Autodesk Inventor part; units mm, degrees
ref_plane "YZ Plane" through (0, 0, 0) normal (1, 0, 0) x (0, 1, 0)
ref_plane "XZ Plane" through (0, 0, 0) normal (0, 1, 0) x (-1, 0, 0)
ref_plane "XY Plane" through (0, 0, 0) normal (0, 0, 1) x (1, 0, 0)
sketch "Sketch1" plane through (0, 0, 0) normal (0, 1, 0) x (-1, 0, 0)
  line L0 (5.5, 6.5) -> (-5.5, 6.5)
  line L1 (-5.5, 6.5) -> (-5.5, -6.5)
  line L2 (-5.5, -6.5) -> (5.5, -6.5)
  line L3 (5.5, -6.5) -> (5.5, 6.5)
  line L4 (0, -9.1) -> (0, 9.1)
  line L5 (-7.7, 0) -> (7.7, 0)
  point P0 (0, 0)
  dimension "d0" = 11
  dimension "d1" = 5.5
  dimension "d2" = 13
  dimension "d3" = 6.5
extrude "Extrusion1" add sketch "Sketch1" along normal blind 5
sketch "Sketch2" plane through (0, 5, 0) normal (0, 1, 0) x (1, 0, 0)
  line L0 (-5.5, -6.5) -> (5.5, -6.5)
  line L1 (-5.24, -6.5) -> (-4.24, -6.5)
  line L2 (-4.24, -6.5) -> (-4.24, 1)
  line L3 (-4.24, 1) -> (-5.24, 1)
  line L4 (-5.24, 1) -> (-5.24, -6.5)
  line L5 (5.24, -6.5) -> (4.24, -6.5)
  line L6 (4.24, -6.5) -> (4.24, 1)
  line L7 (4.24, 1) -> (5.24, 1)
  line L8 (5.24, 1) -> (5.24, -6.5)
  line L9 (5.5, -6.5) -> (5.5, 6.5)
  line L10 (-5.5, 6.5) -> (-5.5, -6.5)
  point P0 (0, 0)
  point P1 (4.74, 1)
  point P2 (4.24, -6.5)
  dimension "d6" = 0.26
  dimension "d7" = 0.26
  dimension "d8" = 1
  dimension "d9" = 1
  dimension "d10" = 7.5
  dimension "d11" = 7.5
extrude "Extrusion2" add sketch "Sketch2" along normal blind 1
sketch "Sketch3" plane through (-5.5, 0, 6.5) normal (0, 0, 1) x (1, 0, 0)
  line L0 (0.95, 4) -> (2.25, 4)
  line L1 (2.25, 4) -> (2.25, 2.7)
  line L2 (2.25, 2.7) -> (0.95, 2.7)
  line L3 (0.95, 2.7) -> (0.95, 4)
  line L4 (3.55, 4) -> (4.85, 4)
  line L5 (4.85, 4) -> (4.85, 2.7)
  line L6 (4.85, 2.7) -> (3.55, 2.7)
  line L7 (3.55, 2.7) -> (3.55, 4)
  line L8 (6.15, 4) -> (7.45, 4)
  line L9 (7.45, 4) -> (7.45, 2.7)
  line L10 (7.45, 2.7) -> (6.15, 2.7)
  line L11 (6.15, 2.7) -> (6.15, 4)
  line L12 (8.75, 4) -> (10.05, 4)
  line L13 (10.05, 4) -> (10.05, 2.7)
  line L14 (10.05, 2.7) -> (8.75, 2.7)
  line L15 (8.75, 2.7) -> (8.75, 4)
  line L16 (0, 0) -> (0, 5)
  line L17 (5.5, 7.2) -> (5.5, -1.2)
  line L18 (1.26, 5) -> (9.74, 5)
  point P0 (5.5, 0)
  point P1 (0.95, 3.35)
  dimension "d14" = 1.3
  dimension "d15" = 1.3
  dimension "d18" = 1.3
  dimension "d19" = 1.3
  dimension "d21" = 1.3
  dimension "d22" = 1.3
  dimension "d23" = 1.3
  dimension "d24" = 0.65
  dimension "d25" = 1.3
  dimension "d26" = 1
extrude "Extrusion3" cut sketch "Sketch3" against normal up to surface (13 mm away)
equation "\"d1\" = 0.5 * d0"
equation "\"d3\" = 0.5 * d2"
equation "\"d7\" = d6"
equation "\"d9\" = d8"
equation "\"d15\" = d14"
equation "\"d18\" = d15"
equation "\"d19\" = d18"
equation "\"d21\" = d19"
equation "\"d22\" = d14"
equation "\"d23\" = d15"
equation "\"d24\" = 0.5 * d19"
equation "\"d25\" = d14"
properties part number "Four-Pin-Shell"
Design review of the part built by this model. Coordinates are the model's own, in mm. A direction names the side the tool comes from. Give positions to 0.01 mm unless a question says otherwise; leave off trailing zeros. Order: outer loops, then holes, each group sorted by start corner. A loop starts at its lowest first (then second) coordinate and runs counter-clockwise, first axis right, second up. Notation, with made-up numbers: (80, 55) -> (130, 55) arc R22 ccw to (130, 66) -> close; hole circle Ø1 at (50.5, 27.25). An arc over 180 degrees is marked (long way). Write each question's results on one line, items separated by ' | '. Start each with the question number.
Q1. Machinability: for faces 5 (the flat face through (-4.24, 5.5, 2.8)), 6 (the flat face through (0, 0, 0)), 7 (the flat face through (-4.7, 5.5, -1)), 8 (the flat face through (4.55, 3, 0)), which of the approach directions +Z, -Z, +X, -X, +Y, -Y give a long, thin tool a straight path to every point of the face, cutting with its end or side? Answer none if there is none.
Q2. Add section B-B on z = 2.25. Give the boundary of the cut face in (x, y).
Q3. Wall thickness on L1, parallel to X at y = 3.1, z = 2.5; L2, parallel to Y at x = -1, z = 0.75; L3, parallel to Z at x = -4.5, y = 5.15: over which ranges is each line inside the solid? List them lowest first. Write a range as from..to.
Q4. Add section C-C on x = -3.5. Give the boundary of the cut face in (y, z), and give its area (3 significant figures).
Q5. Mouldability with a two-part tool opening along Y and no side actions: class faces 1 (the flat face through (5.5, 2, 0)), 2 (the flat face through (-3.25, 3, 0)), 3 (the flat face through (4, 4, 0)), 4 (the flat face through (5, 6, 3)) as +Y half, -Y half, draft (parallel to the pull), parting line (faces both ways), or undercut.
Q6. For pin 1 (0.8 mm diameter, centred on y = 5.5, z = 2, fed in from +X); pin 2 (0.8 mm diameter, centred on x = 5, y = 5.5, fed in from -Z), all flat-tipped, find the tip position at first contact; note any pin that passes through.
Q7. Add section D-D on y = 3.1. Give the boundary of the cut face in (x, z), and give its area (3 significant figures).
Q8. Add section A-A on y = 5.6. Give the boundary of the cut face in (x, z).
Found:
1) face 5: +Z, -Z, +Y | face 6: +Z, -Z, +X, -X, -Y | face 7: -Z, +X, -X, +Y | face 8: +Z, -Z
2) outline: (-5.5, 0) -> (5.5, 0) -> (5.5, 5) -> (5.24, 5) -> (5.24, 6) -> (4.24, 6) -> (4.24, 5) -> (-4.24, 5) -> (-4.24, 6) -> (-5.24, 6) -> (-5.24, 5) -> (-5.5, 5) -> close; hole (-4.55, 2.7) -> (-3.25, 2.7) -> (-3.25, 4) -> (-4.55, 4) -> close; hole (-1.95, 2.7) -> (-0.65, 2.7) -> (-0.65, 4) -> (-1.95, 4) -> close; hole (0.65, 2.7) -> (1.95, 2.7) -> (1.95, 4) -> (0.65, 4) -> close; hole (3.25, 2.7) -> (4.55, 2.7) -> (4.55, 4) -> (3.25, 4) -> close
3) L1: x = -5.5..-4.55, -3.25..-1.95, -0.65..0.65, 1.95..3.25, 4.55..5.5 | L2: y = 0..2.7, 4..5 | L3: z = -1..6.5
4) outline: (0, -6.5) -> (2.7, -6.5) -> (2.7, 6.5) -> (0, 6.5) -> close; (4, -6.5) -> (5, -6.5) -> (5, 6.5) -> (4, 6.5) -> close | area: 48.1 mm2
5) face 1: draft | face 2: undercut | face 3: undercut | face 4: +Y half
6) pin 1: stops at x = 5.24 | pin 2: stops at z = -1
7) outline: (-5.5, -6.5) -> (-4.55, -6.5) -> (-4.55, 6.5) -> (-5.5, 6.5) -> close; (-3.25, -6.5) -> (-1.95, -6.5) -> (-1.95, 6.5) -> (-3.25, 6.5) -> close; (-0.65, -6.5) -> (0.65, -6.5) -> (0.65, 6.5) -> (-0.65, 6.5) -> close; (1.95, -6.5) -> (3.25, -6.5) -> (3.25, 6.5) -> (1.95, 6.5) -> close; (4.55, -6.5) -> (5.5, -6.5) -> (5.5, 6.5) -> (4.55, 6.5) -> close | area: 75.4 mm2
8) outline: (-5.24, -1) -> (-4.24, -1) -> (-4.24, 6.5) -> (-5.24, 6.5) -> close; (4.24, -1) -> (5.24, -1) -> (5.24, 6.5) -> (4.24, 6.5) -> close
